```python
from build123d import *

# Parameters (mm, degrees)
SKETCH_1_W               = 420
SKETCH_1_H               = 420
EXTRUDE_1_DEPTH          = 5
SKETCH_3_W               = 50
SKETCH_3_H               = 10
SKETCH_3_W_2             = 10
SKETCH_3_H_2             = 50
EXTRUDE_2_DEPTH          = 10
SKETCH_4_W               = 200
SKETCH_4_H               = 10
SKETCH_4_W_2             = 10
SKETCH_4_H_2             = 200
EXTRUDE_3_DEPTH          = 10
FILLET_1_R               = 5
SKETCH_5_R               = 2
CUT_EXTRUDE_1_DEPTH      = 422.366823564
SKETCH_6_R               = 2
CUT_EXTRUDE_2_DEPTH      = 375.733238451
CUT_EXTRUDE_3_DEPTH      = 422.366823564
CUT_EXTRUDE_3_DEPTH_BACK = 422.366823564
SKETCH_7_R               = 2
SKETCH_8_R               = 2
CUT_EXTRUDE_4_DEPTH      = 375.733238451
CUT_EXTRUDE_5_DEPTH      = 422.366823564
CUT_EXTRUDE_5_DEPTH_BACK = 422.366823564
SKETCH_9_R               = 2
SKETCH_10_R              = 2
CUT_EXTRUDE_6_DEPTH      = 375.733238451
CUT_EXTRUDE_7_DEPTH      = 422.366823564
CUT_EXTRUDE_7_DEPTH_BACK = 422.366823564
SKETCH_11_R              = 2
SKETCH_12_R              = 2
CUT_EXTRUDE_8_DEPTH      = 375.733238451
SCALE_1_SCALE            = 0.5
SKETCH_13_W              = 210
SKETCH_13_H              = 210
CUT_EXTRUDE_9_DEPTH      = 90
SKETCH_14_W              = 100
SKETCH_14_H              = 100
EXTRUDE_4_DEPTH          = 12
FILLET_2_R               = 12
SKETCH_15_R              = 2
CUT_EXTRUDE_10_DEPTH     = 5


with BuildPart() as part:
    # 草图1 → 凸台-拉伸1 (new body)
    with BuildSketch(Plane.XY):
        Rectangle(SKETCH_1_W, SKETCH_1_H)
    extrude(amount=EXTRUDE_1_DEPTH)

    # 草图3 → 凸台-拉伸2 (add)
    with BuildSketch(Plane(origin=(0, 0, 0), x_dir=(-1, 0, 0), z_dir=(0, 0, -1))):
        with Locations((-130, -205)):
            Rectangle(SKETCH_3_W, SKETCH_3_H)
        with Locations((-205, -130)):
            Rectangle(SKETCH_3_W_2, SKETCH_3_H_2)
        with Locations((-205, 130)):
            Rectangle(SKETCH_3_W_2, SKETCH_3_H_2)
        with Locations((-130, 205)):
            Rectangle(SKETCH_3_W, SKETCH_3_H)
        with Locations((205, 130)):
            Rectangle(SKETCH_3_W_2, SKETCH_3_H_2)
        with Locations((130, 205)):
            Rectangle(SKETCH_3_W, SKETCH_3_H)
        with Locations((205, -130)):
            Rectangle(SKETCH_3_W_2, SKETCH_3_H_2)
        with Locations((130, -205)):
            Rectangle(SKETCH_3_W, SKETCH_3_H)
    extrude(amount=EXTRUDE_2_DEPTH)

    # 草图4 → 凸台-拉伸3 (add)
    with BuildSketch(Plane.XY.offset(5)):
        with Locations((0, -205)):
            Rectangle(SKETCH_4_W, SKETCH_4_H)
        with Locations((205, 0)):
            Rectangle(SKETCH_4_W_2, SKETCH_4_H_2)
        with Locations((0, 205)):
            Rectangle(SKETCH_4_W, SKETCH_4_H)
        with Locations((-205, 0)):
            Rectangle(SKETCH_4_W_2, SKETCH_4_H_2)
    extrude(amount=EXTRUDE_3_DEPTH)

    # 圆角1
    fillet_1_edges = [part.edges().sort_by_distance(p)[0] for p in [
        (-210, 0, 15),
        (-200, 0, 15),
        (0, -210, 15),
        (0, -200, 15),
        (0, 200, 15),
        (0, 210, 15),
        (200, 0, 15),
        (210, 0, 15),
        (200, -130, -10),
        (210, -130, -10),
        (130, 210, -10),
        (130, 200, -10),
        (200, 130, -10),
        (210, 130, -10),
        (-130, -200, -10),
        (-130, -210, -10),
        (-130, 210, -10),
        (-130, 200, -10),
        (-210, 130, -10),
        (-200, 130, -10),
        (-210, -130, -10),
        (-200, -130, -10),
        (130, -200, -10),
        (130, -210, -10),
    ]]
    fillet(fillet_1_edges, radius=FILLET_1_R - 0.0001)  # a hair under: the kernel refuses the full size

    # 草图5 → 切除-拉伸1 (cut, through all)
    with BuildSketch(Plane(origin=(0, 155, 0), x_dir=(1, 0, 0), z_dir=(0, 1, 0))):
        with Locations(Location((205, 5, 0), (0, 0, 270))):
            Circle(SKETCH_5_R)
    extrude(amount=-CUT_EXTRUDE_1_DEPTH, mode=Mode.SUBTRACT)

    # 草图6 → 切除-拉伸2 (cut, through all)
    with BuildSketch(Plane(origin=(0, 100, 0), x_dir=(1, 0, 0), z_dir=(0, 1, 0))):
        with Locations(Location((205, -10, 0), (0, 0, 270))):
            Circle(SKETCH_6_R)
    extrude(amount=-CUT_EXTRUDE_2_DEPTH, mode=Mode.SUBTRACT)

    # 草图7 → 切除-拉伸3 (cut, two sides: drawn at the far end of the back side and taken through both)
    with BuildSketch(Plane(origin=(155, 0, 0), x_dir=(0, 0, -1), z_dir=(1, 0, 0)).offset(-CUT_EXTRUDE_3_DEPTH_BACK)):
        with Locations((5, -205)):
            Circle(SKETCH_7_R)
    extrude(amount=CUT_EXTRUDE_3_DEPTH + CUT_EXTRUDE_3_DEPTH_BACK, mode=Mode.SUBTRACT)

    # 草图8 → 切除-拉伸4 (cut, through all)
    with BuildSketch(Plane(origin=(100, 0, 0), x_dir=(0, 0, -1), z_dir=(1, 0, 0))):
        with Locations((-10, -205)):
            Circle(SKETCH_8_R)
    extrude(amount=-CUT_EXTRUDE_4_DEPTH, mode=Mode.SUBTRACT)

    # 草图9 → 切除-拉伸5 (cut, two sides: drawn at the far end of the back side and taken through both)
    with BuildSketch(Plane.XZ.offset(155).offset(-CUT_EXTRUDE_5_DEPTH_BACK)):
        with Locations((-205, -5)):
            Circle(SKETCH_9_R)
    extrude(amount=CUT_EXTRUDE_5_DEPTH + CUT_EXTRUDE_5_DEPTH_BACK, mode=Mode.SUBTRACT)

    # 草图10 → 切除-拉伸6 (cut, through all)
    with BuildSketch(Plane.XZ.offset(100)):
        with Locations(Location((-205, 10, 0), (0, 0, 270))):
            Circle(SKETCH_10_R)
    extrude(amount=-CUT_EXTRUDE_6_DEPTH, mode=Mode.SUBTRACT)

    # 草图11 → 切除-拉伸7 (cut, two sides: drawn at the far end of the back side and taken through both)
    with BuildSketch(Plane.ZY.offset(155).offset(-CUT_EXTRUDE_7_DEPTH_BACK)):
        with Locations(Location((-5, 205, 0), (0, 0, 270))):
            Circle(SKETCH_11_R)
    extrude(amount=CUT_EXTRUDE_7_DEPTH + CUT_EXTRUDE_7_DEPTH_BACK, mode=Mode.SUBTRACT)

    # 草图12 → 切除-拉伸8 (cut, through all)
    with BuildSketch(Plane.ZY.offset(100)):
        with Locations((10, 205)):
            Circle(SKETCH_12_R)
    extrude(amount=-CUT_EXTRUDE_8_DEPTH, mode=Mode.SUBTRACT)


with BuildPart() as part_1:
    # 缩放比例1: scaled about (0, 0, 0)
    add(part.part.scale(SCALE_1_SCALE))

    # 草图13 → 切除-拉伸9 (cut)
    with BuildSketch(Plane(origin=(0, 0, 0), x_dir=(-1, 0, 0), z_dir=(0, 0, -1))):
        Rectangle(SKETCH_13_W, SKETCH_13_H)
    extrude(amount=CUT_EXTRUDE_9_DEPTH, mode=Mode.SUBTRACT)

    # 草图14 → 凸台-拉伸4 (add)
    with BuildSketch(Plane(origin=(0, 0, 0), x_dir=(-1, 0, 0), z_dir=(0, 0, -1))):
        Rectangle(SKETCH_14_W, SKETCH_14_H)
    extrude(amount=EXTRUDE_4_DEPTH)

    # 圆角2
    fillet_2_edges = [part_1.edges().sort_by_distance(p)[0] for p in [
        (50, 0, 0),
        (0, -50, 0),
        (-50, 0, 0),
        (0, 50, 0),
    ]]
    fillet(fillet_2_edges, radius=FILLET_2_R - 0.0001)  # a hair under: the kernel refuses the full size

    # 草图15 → 切除-拉伸10 (cut)
    with BuildSketch(Plane(origin=(0, 0, -12), x_dir=(-1, 0, 0), z_dir=(0, 0, -1))):
        with Locations((-35, 35)):
            Circle(SKETCH_15_R)
        with Locations((35, 35)):
            Circle(SKETCH_15_R)
        with Locations((-35, -35)):
            Circle(SKETCH_15_R)
        with Locations((35, -35)):
            Circle(SKETCH_15_R)
    extrude(amount=-CUT_EXTRUDE_10_DEPTH, mode=Mode.SUBTRACT)


solid = part_1.part
```
Verification items for the finished model (mm, model axes). A direction names the side the tool comes from. Coordinates: 2 decimals unless noted, no trailing zeros. Write each loop counter-clockwise with the first axis right and the second up, starting at its lowest first coordinate (ties: lowest second). Pieces come first, ordered by that corner, then holes. Notation, with made-up numbers: (74, 56) - (122, 56) arc R29 cw to (122, 80) - close; hole circle Ø3 at (79, 12). An arc over 180 degrees is marked (long way). Write item = value, one per line.
Q1. Cross-section at A-A (x = -44.5). Give the number of separate pieces and of enclosed holes in the cut face, plus the area to 3 significant figures.
Answer:
separate_pieces = 1
enclosed_holes = 2
area = 1,830 mm²
Q2. Access from +Z, -Z, +X, -X, +Y, -Y to the whole of each face (thin tool, end or side, straight path). Record for faces 1 (the face through (-102.54, -50, 3.85)), 2 (the face through (50, 102.46, 3.85)), 3 (the face through (-50, 102.46, 3.85)).
Answer:
face_1 = +Z, +X, -X, -Y
face_2 = +Z, +X, +Y, -Y
face_3 = +Z, -X, +Y, -Y
Q3. Mould release check, pull along Y, two halves, no side actions. Record for faces 4 (the face through (-1, 1, 2.5)), 5 (the face through (105, -1, 2)), 6 (the face through (-1, -105, 2)), 7 (the face through (-102.54, 50, 3.85)): released by +Y, released by -Y, zero draft, split by the parting line, or undercut.
Answer:
face_4 = undercut
face_5 = zero draft
face_6 = released by -Y
face_7 = released by +Y
Q4. Material ranges on L1, parallel to Y at x = 16, z = 5; L2, parallel to X at y = -14.5, z = 2.75, recorded low to high. Write a range as from..to.
Answer:
L1 = -105..-103.5, -101.5..-100, 100..101.5, 103.5..105
L2 = -105..-100, 100..105
Q5. Cross-section at B-B (x = -76). Enter the section's corners in (y, z), plus the area to 3 significant figures.
Answer:
outline = (-105, 0) - (105, 0) - (105, 2.5) - (-105, 2.5) - close
area = 525 mm²
Q6. Go/stop test with flat-tipped pins: pin 1 Ø6 at (x, y) = (-54.5, -33.5) entering from -Z; pin 2 Ø2.5 at (y, z) = (-102.5, 4.5) entering from +X; pin 3 Ø2 at (y, z) = (-37, -8) entering from -X; pin 4 Ø4.5 at (x, y) = (-35, -35) entering from -Z. Record where each tip stops, or that it passes through.
Answer:
pin_1 = -6.19
pin_2 = 50
pin_3 = -51.09
pin_4 = -12
